Verification items for the finished model (mm, model axes). A direction names the side the tool comes from. Give positions to 0.01 mm unless a question says otherwise; leave off trailing zeros. Order: outer loops, then holes, each group sorted by start corner. A loop starts at its lowest first (then second) coordinate and runs counter-clockwise, first axis right, second up. Notation, with made-up numbers: (53, 68.5) -> (104, 68.5) arc R32 ccw to (104, 103.5) -> close; hole circle Ø2 at (76, -11.5). An arc over 180 degrees is marked (long way). Write each question's results on one line, items separated by ' | '. Start each with the question number.
1. Depth check by flat-ended pin: pin 1 Ø2 at (y, z) = (3, 1.5) entering from +X; pin 2 Ø2.5 at (x, y) = (71.5, 2) entering from +Z; pin 3 Ø1.2 at (y, z) = (-0.5, 4.5) entering from -X. Enter the tip coordinate at first touch or a pass-through.
2. Cross-section at B-B, the plane y = 0. State how many separate pieces and enclosed holes the cut face has, then the cut area to 3 significant figures.
3. Set-up check for faces 4 (the face through (67, 0, 3.1)), 5 (the face through (3, 0, 7)), 6 (the face through (67, 0, 6.9)), 7 (the face through (-5, 0, 1)): record each of +Z, -Z, +X, -X, +Y, -Y from which the full face is reachable in a straight line by a thin tool's end or side.
4. Cross-section at A-A, the plane z = 4.5. Enter the section's corners in (x, y).
5. Material ranges on L1, parallel to X at y = 0, z = 1.7; L2, parallel to Y at x = 70, z = 5.85; L3, parallel to Z at x = 1, y = -3.75, recorded low to high. Write a range as from..to.
6. Mould release check, pull along Z, two halves, no side actions. Record for faces 1 (the face through (64.5, 0, 8)), 2 (the face through (74.634, -0.102, 3.235)), 3 (the face through (-4.634, -0.102, 2.865)): +Z half, -Z half, draft (parallel to the pull), parting line (faces both ways), or undercut.
from build123d import *

# Parameters (mm, degrees)
SKETCH1_R           = 1.6
BOSS_EXTRUDE1_DEPTH = 10
CUT_EXTRUDE1_START  = -7
CUT_EXTRUDE1_DEPTH  = 4
CHAMFER1_SIZE       = 0.5
CUT_EXTRUDE2_START  = -3.1
CUT_EXTRUDE2_DEPTH  = 3.1
CUT_EXTRUDE3_START  = -6.9
CUT_EXTRUDE3_DEPTH  = 3.1
CHAMFER2_SIZE       = 0.5


with BuildPart() as part:
    # Sketch1 → Boss-Extrude1 (new body)
    with BuildSketch(Plane.XY):
        with BuildLine():
            Line((0, 5), (70, 5))
            ThreePointArc((70, 5), (75, 0), (70, -5))
            Line((70, -5), (0, -5))
            ThreePointArc((0, -5), (-5, 0), (0, 5))
        make_face()
        Circle(SKETCH1_R, mode=Mode.SUBTRACT)
        with Locations((70, 0)):
            Circle(SKETCH1_R, mode=Mode.SUBTRACT)
    extrude(amount=BOSS_EXTRUDE1_DEPTH)

    # Sketch2 → Cut-Extrude1 (cut)
    with BuildSketch(Plane.XY.offset(10).offset(CUT_EXTRUDE1_START)):
        with BuildLine():
            Line((5.5, 5), (5.5, -5))
            Line((5.5, -5), (0, -5))
            ThreePointArc((0, -5), (-5, 0), (0, 5))
            Line((0, 5), (5.5, 5))
        make_face()
    extrude(amount=CUT_EXTRUDE1_DEPTH, mode=Mode.SUBTRACT)

    # Chamfer1
    chamfer1_edges = [part.edges().sort_by_distance(p)[0] for p in [
        (75, 0, 10),
        (-1.6, 0, 0),
        (-1.6, 0, 10),
        (35, 5, 10),
        (68.4, 0, 0),
        (68.4, 0, 10),
        (-1.6, 0, 3),
        (2.75, 5, 3),
        (5.5, 5, 5),
        (2.75, -5, 3),
        (5.5, -5, 5),
        (-5, 0, 3),
        (-1.6, 0, 7),
        (2.75, 5, 7),
        (-5, 0, 7),
        (2.75, -5, 7),
        (-5, 0, 10),
        (35, 5, 0),
        (75, 0, 0),
        (35, -5, 0),
        (-5, 0, 0),
        (35, -5, 10),
    ]]
    chamfer(chamfer1_edges, length=CHAMFER1_SIZE)

    # Sketch3 → Cut-Extrude2 (cut)
    with BuildSketch(Plane.XY.offset(10).offset(CUT_EXTRUDE2_START)):
        with BuildLine():
            Line((64.5, 5), (64.5, -5))
            Line((64.5, -5), (70, -5))
            ThreePointArc((70, -5), (75, 0), (70, 5))
            Line((70, 5), (64.5, 5))
        make_face()
    extrude(amount=CUT_EXTRUDE2_DEPTH, mode=Mode.SUBTRACT)

    # Sketch4 → Cut-Extrude3 (cut)
    with BuildSketch(Plane.XY.offset(6.9).offset(CUT_EXTRUDE3_START)):
        with BuildLine():
            Line((64.5, 5), (64.5, -5))
            Line((64.5, -5), (70, -5))
            ThreePointArc((70, -5), (75, 0), (70, 5))
            Line((70, 5), (64.5, 5))
        make_face()
    extrude(amount=CUT_EXTRUDE3_DEPTH, mode=Mode.SUBTRACT)

    # Chamfer2
    # the kernel refuses this chamfer: 0.5 mm, written as the material it takes off along each edge
    with BuildSketch(Plane(origin=(70, 0, 6.9), x_dir=(1, 0, 0), z_dir=(0, 1, 0))) as chamfer2_piece_1:
        Polygon((1.6 + CHAMFER2_SIZE, 0), (1.6, CHAMFER2_SIZE), (1.6, 0), align=None)
    revolve(axis=Axis((70, 0, 6.9), (0, 0, -1)), mode=Mode.SUBTRACT)
    with BuildSketch(Plane(origin=(70, 0, 3.1), x_dir=(1, 0, 0), z_dir=(0, 1, 0))) as chamfer2_piece_2:
        Polygon((1.6 + CHAMFER2_SIZE, 0), (1.6, -CHAMFER2_SIZE), (1.6, 0), align=None)
    revolve(axis=Axis((70, 0, 3.1), (0, 0, -1)), mode=Mode.SUBTRACT)
    with BuildSketch(Plane(origin=(64.5, -5, -0.785841494), x_dir=(0.0274958766105822, 0.999621916911297, 0), z_dir=(0, 0, 1)), Plane(origin=(64.5, 5, -0.785841494), x_dir=(-0.9996219169112968, 0.02749587661058574, 0), z_dir=(0, 0, 1)), Plane(origin=(64.5, -5, 6.9), x_dir=(0.0274958766105822, 0.999621916911297, 0), z_dir=(0, 0, 1)), Plane(origin=(64.5, 5, 6.9), x_dir=(-0.9996219169112973, 0.027495876610566763, 0), z_dir=(0, 0, 1))) as chamfer2_piece_3:
        Polygon((CHAMFER2_SIZE * 0.999621916911, CHAMFER2_SIZE * 0.0274958766106), (-CHAMFER2_SIZE * 0.0274958766106, CHAMFER2_SIZE * 0.999621916911), (0, 0), align=None)
    extrude(amount=3.885841494, mode=Mode.SUBTRACT)
    with BuildSketch(Plane(origin=(64.5, 5.785841494, 0), x_dir=(0.027495876610582174, 0, 0.9996219169112968), z_dir=(0, -1, 0))) as chamfer2_piece_4:
        Polygon((CHAMFER2_SIZE * 0.999621916911, CHAMFER2_SIZE * 0.0274958766106), (-CHAMFER2_SIZE * 0.0274958766106, CHAMFER2_SIZE * 0.999621916911), (0, 0), align=None)
    extrude(amount=11.571682988, mode=Mode.SUBTRACT)
    with BuildSketch(Plane(origin=(64.5, -5, 3.1), x_dir=(0, 0.9996219169112968, -0.027495876610586462), z_dir=(1, 0, 0)), Plane(origin=(70, 5, 6.9), x_dir=(0, 0.027495876610585647, -0.9996219169112968), z_dir=(-1, 0, 0))) as chamfer2_piece_5:
        Polygon((CHAMFER2_SIZE * 0.999621916911, CHAMFER2_SIZE * 0.0274958766106), (-CHAMFER2_SIZE * 0.0274958766106, CHAMFER2_SIZE * 0.999621916911), (0, 0), align=None)
    extrude(amount=5.5, mode=Mode.SUBTRACT)
    with BuildSketch(Plane(origin=(70, 0, 3.1), x_dir=(0, -1, 0), z_dir=(-1, 0, 0))) as chamfer2_piece_6:
        Polygon((5, CHAMFER2_SIZE), (5 - CHAMFER2_SIZE, 0), (5, 0), align=None)
    revolve(axis=Axis((70, 0, 3.1), (0, 0, 1)), revolution_arc=180, mode=Mode.SUBTRACT)
    with BuildSketch(Plane(origin=(70, 5, 3.1), x_dir=(0, 0.027495876610585623, 0.9996219169112968), z_dir=(-1, 0, 0)), Plane(origin=(64.5, -5, 6.9), x_dir=(0, 0.9996219169112968, 0.0274958766105856), z_dir=(1, 0, 0))) as chamfer2_piece_7:
        Polygon((CHAMFER2_SIZE * 0.999621916911, -CHAMFER2_SIZE * 0.0274958766106), (-CHAMFER2_SIZE * 0.0274958766106, -CHAMFER2_SIZE * 0.999621916911), (0, 0), align=None)
    extrude(amount=5.5, mode=Mode.SUBTRACT)
    with BuildSketch(Plane(origin=(64.5, 5.785841494, 10), x_dir=(0.0274958766105822, 0, -0.999621916911297), z_dir=(0, -1, 0))) as chamfer2_piece_8:
        Polygon((CHAMFER2_SIZE * 0.999621916911, -CHAMFER2_SIZE * 0.0274958766106), (-CHAMFER2_SIZE * 0.0274958766106, -CHAMFER2_SIZE * 0.999621916911), (0, 0), align=None)
    extrude(amount=11.571682988, mode=Mode.SUBTRACT)
    with BuildSketch(Plane(origin=(70, 0, 6.9), x_dir=(0, -1, 0), z_dir=(-1, 0, 0))) as chamfer2_piece_9:
        Polygon((5, -CHAMFER2_SIZE), (5 - CHAMFER2_SIZE, 0), (5, 0), align=None)
    revolve(axis=Axis((70, 0, 6.9), (0, 0, 1)), revolution_arc=180, mode=Mode.SUBTRACT)
    with BuildSketch(Plane(origin=(64.5, -5, -0.785841494), x_dir=(0.0274958766105822, 0.999621916911297, 0), z_dir=(0, 0, 1))) as chamfer2_piece_10a_section:
        Polygon((CHAMFER2_SIZE * 0.999621916911, CHAMFER2_SIZE * 0.0274958766106), (-CHAMFER2_SIZE * 0.0274958766106, CHAMFER2_SIZE * 0.999621916911), (0, 0), align=None)
    chamfer2_piece_10a = extrude(amount=5.171682988, mode=Mode.PRIVATE)
    chamfer2_piece_10a = split(chamfer2_piece_10a, bisect_by=Plane(origin=(64.335103187, -4.835103187, 3.1), z_dir=(0, 0, 1)), keep=Keep.TOP, mode=Mode.PRIVATE)
    with BuildSketch(Plane(origin=(63.214158506, -5, 3.1), x_dir=(0, 0.9996219169112968, -0.02749587661058651), z_dir=(1, 0, 0))) as chamfer2_piece_10b_section:
        Polygon((CHAMFER2_SIZE * 0.999621916911, CHAMFER2_SIZE * 0.0274958766106), (-CHAMFER2_SIZE * 0.0274958766106, CHAMFER2_SIZE * 0.999621916911), (0, 0), align=None)
    chamfer2_piece_10b = extrude(amount=6.785841494, mode=Mode.PRIVATE)
    chamfer2_piece_10b = split(chamfer2_piece_10b, bisect_by=Plane(origin=(64.5, -4.835103187, 3.264896813), z_dir=(-1, 0, 0)), keep=Keep.TOP, mode=Mode.PRIVATE)
    chamfer2_piece_10 = chamfer2_piece_10a & chamfer2_piece_10b
    add(chamfer2_piece_10, mode=Mode.SUBTRACT)
    with BuildSketch(Plane(origin=(64.5, 5, -0.785841494), x_dir=(-0.9996219169112968, 0.02749587661058574, 0), z_dir=(0, 0, 1))) as chamfer2_piece_11a_section:
        Polygon((CHAMFER2_SIZE * 0.999621916911, CHAMFER2_SIZE * 0.0274958766106), (-CHAMFER2_SIZE * 0.0274958766106, CHAMFER2_SIZE * 0.999621916911), (0, 0), align=None)
    chamfer2_piece_11a = extrude(amount=5.171682988, mode=Mode.PRIVATE)
    chamfer2_piece_11a = split(chamfer2_piece_11a, bisect_by=Plane(origin=(64.335103187, 4.835103187, 3.1), z_dir=(0, 0, 1)), keep=Keep.TOP, mode=Mode.PRIVATE)
    with BuildSketch(Plane(origin=(70, 5, 3.1), x_dir=(0, 0.027495876610585623, 0.9996219169112968), z_dir=(-1, 0, 0))) as chamfer2_piece_11b_section:
        Polygon((CHAMFER2_SIZE * 0.999621916911, -CHAMFER2_SIZE * 0.0274958766106), (-CHAMFER2_SIZE * 0.0274958766106, -CHAMFER2_SIZE * 0.999621916911), (0, 0), align=None)
    chamfer2_piece_11b = extrude(amount=6.785841494, mode=Mode.PRIVATE)
    chamfer2_piece_11b = split(chamfer2_piece_11b, bisect_by=Plane(origin=(64.5, 4.835103187, 3.264896813), z_dir=(-1, 0, 0)), keep=Keep.TOP, mode=Mode.PRIVATE)
    chamfer2_piece_11 = chamfer2_piece_11a & chamfer2_piece_11b
    add(chamfer2_piece_11, mode=Mode.SUBTRACT)
    with BuildSketch(Plane(origin=(63.214158506, -5, 6.9), x_dir=(0, 0.9996219169112968, 0.027495876610585647), z_dir=(1, 0, 0))) as chamfer2_piece_12a_section:
        Polygon((CHAMFER2_SIZE * 0.999621916911, -CHAMFER2_SIZE * 0.0274958766106), (-CHAMFER2_SIZE * 0.0274958766106, -CHAMFER2_SIZE * 0.999621916911), (0, 0), align=None)
    chamfer2_piece_12a = extrude(amount=6.785841494, mode=Mode.PRIVATE)
    chamfer2_piece_12a = split(chamfer2_piece_12a, bisect_by=Plane(origin=(64.5, -4.835103187, 6.735103187), z_dir=(-1, 0, 0)), keep=Keep.TOP, mode=Mode.PRIVATE)
    with BuildSketch(Plane(origin=(64.5, -5, 5.614158506), x_dir=(0.0274958766105822, 0.999621916911297, 0), z_dir=(0, 0, 1))) as chamfer2_piece_12b_section:
        Polygon((CHAMFER2_SIZE * 0.999621916911, CHAMFER2_SIZE * 0.0274958766106), (-CHAMFER2_SIZE * 0.0274958766106, CHAMFER2_SIZE * 0.999621916911), (0, 0), align=None)
    chamfer2_piece_12b = extrude(amount=5.171682988, mode=Mode.PRIVATE)
    chamfer2_piece_12b = split(chamfer2_piece_12b, bisect_by=Plane(origin=(64.335103187, -4.835103187, 6.9), z_dir=(0, 0, -1)), keep=Keep.TOP, mode=Mode.PRIVATE)
    chamfer2_piece_12 = chamfer2_piece_12a & chamfer2_piece_12b
    add(chamfer2_piece_12, mode=Mode.SUBTRACT)
    with BuildSketch(Plane(origin=(70, 5, 6.9), x_dir=(0, 0.027495876610585647, -0.9996219169112968), z_dir=(-1, 0, 0))) as chamfer2_piece_13a_section:
        Polygon((CHAMFER2_SIZE * 0.999621916911, CHAMFER2_SIZE * 0.0274958766106), (-CHAMFER2_SIZE * 0.0274958766106, CHAMFER2_SIZE * 0.999621916911), (0, 0), align=None)
    chamfer2_piece_13a = extrude(amount=6.785841494, mode=Mode.PRIVATE)
    chamfer2_piece_13a = split(chamfer2_piece_13a, bisect_by=Plane(origin=(64.5, 4.835103187, 6.735103187), z_dir=(-1, 0, 0)), keep=Keep.TOP, mode=Mode.PRIVATE)
    with BuildSketch(Plane(origin=(64.5, 5, 5.614158506), x_dir=(-0.9996219169112968, 0.02749587661058574, 0), z_dir=(0, 0, 1))) as chamfer2_piece_13b_section:
        Polygon((CHAMFER2_SIZE * 0.999621916911, CHAMFER2_SIZE * 0.0274958766106), (-CHAMFER2_SIZE * 0.0274958766106, CHAMFER2_SIZE * 0.999621916911), (0, 0), align=None)
    chamfer2_piece_13b = extrude(amount=5.171682988, mode=Mode.PRIVATE)
    chamfer2_piece_13b = split(chamfer2_piece_13b, bisect_by=Plane(origin=(64.335103187, 4.835103187, 6.9), z_dir=(0, 0, -1)), keep=Keep.TOP, mode=Mode.PRIVATE)
    chamfer2_piece_13 = chamfer2_piece_13a & chamfer2_piece_13b
    add(chamfer2_piece_13, mode=Mode.SUBTRACT)


solid = part.part
Results below:
1) pin 1: stops at x = 64.5 | pin 2: stops at z = 6.9 | pin 3: stops at x = 5.5
2) separate pieces: 4 | enclosed holes: 0 | area: 659 mm²
3) face 4: -Z, +X, +Y, -Y | face 5: -X, +Y, -Y | face 6: +Z, +X, +Y, -Y | face 7: +Z, -Z, -X
4) outline: (5.5, -4.5) -> (6, -5) -> (70, -5) arc R5 ccw to (70, 5) -> (6, 5) -> (5.5, 4.5) -> close; hole circle Ø3.2 at (70, 0)
5) L1: x = -5..-1.6, 1.6..64.5 | L2: y = -5..-1.6, 1.6..5 | L3: z = 0..3, 7..10
6) face 1: draft | face 2: -Z half | face 3: undercut
